```python
from build123d import *

# Parameters (mm, degrees)
SKETCH_1_W      = 183
SKETCH_1_H      = 187
EXTRUDE_1_DEPTH = 80
SKETCH_3_W      = 5
SKETCH_3_H      = 1


with BuildPart() as part:
    # 草图1 → 拉伸1 (new body)
    with BuildSketch(Plane(origin=(0, 0, 0), x_dir=(1, 0, 0), z_dir=(0, 1, 0))):
        with Locations((91.5, 93.5)):
            Rectangle(SKETCH_1_W, SKETCH_1_H)
    extrude(amount=EXTRUDE_1_DEPTH)

    # 扫描1: sweep along a path in 草图4
    with BuildLine(Plane.ZY.offset(-4)) as sweep_1_path:
        Line((-177, 80), (-177, 85))
        Line((-177, 85), (-167, 85))
    # 草图3 → 扫描1 (sweep)
    with BuildSketch(Plane(origin=(0, 80, 0), x_dir=(-1, 0, 0), z_dir=(0, 1, 0))):
        with Locations((-6.5, -176.5)):
            Rectangle(SKETCH_3_W, SKETCH_3_H)
    sweep_1 = sweep(path=sweep_1_path.line, transition=Transition.RIGHT)

    # 镜向2: 扫描1 across plane
    add(sweep_1.mirror(Plane.ZY.offset(-91.5)))


solid = part.part
```
Verification items for the finished model (mm, model axes). A direction names the side the tool comes from. Coordinates: 2 decimals unless noted, no trailing zeros. Write each loop counter-clockwise with the first axis right and the second up, starting at its lowest first coordinate (ties: lowest second). Pieces come first, ordered by that corner, then holes. Notation, with made-up numbers: M -37.75,79.5 L -15.75,79.5 A23 ccw -15.75,108.5 Z; hole C 7.5,-37.5 d11. An arc over 180 degrees is marked long. One line per item, written item: value.
Item 1: Section check B-B, the plane x = 24. Record the boundary of the cut face in (y, z), plus the area to 3 significant figures.
Check sheet entries:
outline: M 0,-187 L 80,-187 L 80,0 L 0,0 Z
area: 15,000 mm^2
Item 2: Section check A-A, the plane z = -119. Record the boundary of the cut face in (x, y), plus the area to 3 significant figures.
Check sheet entries:
outline: M 0,0 L 183,0 L 183,80 L 0,80 Z
area: 14,600 mm^2
Item 3: Mould release check, pull along Y, two halves, no side actions. Record for faces 6 (the flat face through (7, 83, -177)), 7 (the flat face through (90, 0, -95)), 8 (the flat face through (7, 85, -172)), 9 (the flat face through (6, 84, -171)): pulls with the +Y half, pulls with the -Y half, needs draft (parallel to the pull), parting line crosses it, or undercut.
Check sheet entries:
face 6: needs draft
face 7: pulls with the -Y half
face 8: pulls with the +Y half
face 9: undercut
Item 4: Scan line: line 1 along Y through (x, z) = (108, -45). Record every from-to range of solid material in increasing order.
Check sheet entries:
line 1: y = 0 to 80
Item 5: Gauge pin test, flat ends, axial feed: pin 1 Ø4 at (y, z) = (83.5, -172.5) entering from -X; pin 2 Ø1.2 at (x, y) = (176.5, 83) entering from +Z; pin 3 Ø12 at (x, z) = (88, -56) entering from +Y; pin 4 Ø2.5 at (y, z) = (82.5, -171) entering from +X. Record the tip position at first contact, or that the pin passes through.
Check sheet entries:
pin 1: stops at x = 4
pin 2: stops at z = -176
pin 3: stops at y = 80
pin 4: passes through
Item 6: Access from +Z, -Z, +X, -X, +Y, -Y to the whole of each face (thin tool, end or side, straight path). Record for faces 1 (the flat face through (176, 83, -177)), 2 (the flat face through (4, 84.2, -173.1)), 3 (the flat face through (174, 84.2, -173.5)), 4 (the flat face through (179, 84.2, -173.1)), 5 (the flat face through (177, 84, -171)).
Check sheet entries:
face 1: -Z, +X, -X, +Y
face 2: +Z, -Z, -X, +Y
face 3: +Z, -Z, +Y
face 4: +Z, -Z, +X, +Y
face 5: +Z, +X, -X
